Here's how the part is built. I have some questions about the finished solid (model axes, mm). A direction names the side the tool comes from. Round coordinates to 2 decimals unless told otherwise and drop trailing zeros. Use one line per item in the form item = value. Start each with the question number.
Item 1: Thinking about a two-plate mould opening in Z: for faces 1 (the face through (-9, -6, 31.75)), 2 (the face through (0, 0, 0)), 3 (the face through (-2.9, -13, 33.4)), which applies, released by +Z, released by -Z, zero draft, split by the parting line, or undercut?
Item 2: For faces 4 (the face through (-15.12, -11.59, 6.44)), 5 (the face through (6, -6, 34.925)), which set-ups out of +Z, -Z, +X, -X, +Y, -Y let a thin tool reach every point of the face, with its end or its side?
Item 3: If I drill on L1, parallel to Z at x = -7.5, y = 7 (3 decimals); L2, parallel to Z at x = -2, y = 13 (3 decimals); L3, parallel to Z at x = -11, y = -2 (3 decimals), over which ranges is the centre line in solid material (lowest first)? Write a range as [from, to].
Item 4: If we section it at A-A (y = 7.5): State how many separate pieces and enclosed holes the cut face has, then the cut area to 3 significant figures.
Item 5: I'm going to push flat-ended pins straight in: pin 1 Ø3 at (x, z) = (6, 42.5) entering from -Y; pin 2 Ø8 at (x, y) = (3.5, 2) entering from +Z; pin 3 Ø3 at (x, z) = (-3, 40) entering from -Y; pin 4 Ø2 at (x, y) = (-15, -13) entering from +Z. Where does each tip first touch, or does it pass through?
```python
from build123d import *


with BuildPart() as f1:
    # F0 (on Front) → F1 (revolve)
    with BuildSketch(Plane.XZ):
        with BuildLine():
            Line((0, 50.8), (0, 34.925))
            Line((0, 34.925), (6.7313371377, 34.925))
            add(Edge.make_bspline(
                [(6.7313371377, 34.925), (9.1660192998, 36.584243404), (12.1811256362, 40.5329028803), (9.7038379806, 47.230680767), (6.3139233711, 50.4087846074), (4.754697213, 50.6305893646), (0, 50.8)],
                knots=[0, 0, 0, 0, 0.277452726, 0.5363338254, 0.7326009529, 1, 1, 1, 1], degree=3))
        make_face()
        Polygon((0, 34.925), (0, 31.75), (9.525, 31.75), (13.320277445, 31.75), (13.320277445, 34.925), (6.7313371377, 34.925), align=None)
        with BuildLine():
            Line((0, 31.75), (0, 0))
            Line((0, 0), (19.05, 0))
            Line((19.05, 0), (19.05, 12.7))
            add(Edge.make_bspline(
                [(19.05, 12.7), (15.6445959161, 14.8300528587), (9.037378424, 18.1241412945), (7.0251417677, 23.6118438651), (6.2528101904, 29.2835176444), (9.525, 31.75)],
                knots=[0, 0, 0, 0, 0.3900175878, 0.6631477467, 1, 1, 1, 1], degree=3))
            Line((9.525, 31.75), (0, 31.75))
        make_face()
    revolve(axis=Axis((0, 0, 25.4), (0, 0, 1)))


solid = f1.part
```
Values found:
q1.face_1 = undercut
q1.face_2 = released by -Z
q1.face_3 = zero draft
q2.face_4 = +Z, -Z
q2.face_5 = none
q3.L1 = [0, 18.303], [31.75, 34.925], [38.618, 45.261]
q3.L2 = [0, 16.233], [31.75, 34.925]
q3.L3 = [0, 17.568], [31.75, 34.925]
q4.separate_pieces = 3
q4.enclosed_holes = 0
q4.area = 874 mm2
q5.pin_1 = -10.04
q5.pin_2 = 50.8
q5.pin_3 = -10.84
q5.pin_4 = 12.82
